Autodesk Inventor part; units mm, degrees
ref_plane "YZ Plane" through (0, 0, 0) normal (1, 0, 0) x (0, 1, 0)
ref_plane "XZ Plane" through (0, 0, 0) normal (0, 1, 0) x (-1, 0, 0)
ref_plane "XY Plane" through (0, 0, 0) normal (0, 0, 1) x (1, 0, 0)
sketch "スケッチ1" plane through (0, 0, 0) normal (0, 0, 1) x (1, 0, 0)
  circle A0 centre (0, 0) radius 25
  dimension "d0" = 50
extrude "押し出し1" add sketch "スケッチ1" along normal blind 15
sketch "スケッチ2" plane through (0, 0, 0) normal (0, 0, -1) x (-1, 0, 0)
  circle A0 centre (0, 0) radius 10
  circle A1 centre (0, 0) radius 21
  dimension "d3" = 20
  dimension "d6" = 42
extrude "押し出し2" cut sketch "スケッチ2" against normal blind 13 contours A0
extrude "押し出し3" cut sketch "スケッチ2" against normal blind 3
chamfer "面取り1" distance 2 angle 45 1 edges at (21, 0, 0)
chamfer "面取り2" distance 2 angle 45 1 edges at (10, 0, 3)
properties part number "storage"
Model file for the job. Use its own axes, mm. A direction names the side the tool comes from. Round coordinates to 2 decimals unless told otherwise and drop trailing zeros. Write each loop counter-clockwise with the first axis right and the second up, starting at its lowest first coordinate (ties: lowest second). Pieces come first, ordered by that corner, then holes. Notation, with made-up numbers: (17, 18.25) -> (29, 18.25) arc R22 ccw to (29, 44.25) -> close; hole circle Ø8 at (19, 74.25). An arc over 180 degrees is marked (long way). Answer as CSV lines item,"result".
1. Pin check, flat tips, straight feed: pin 1 Ø1 at (x, y) = (12, -14) entering from -Z; pin 2 Ø6 at (y, z) = (-10.5, 10.5) entering from +X; pin 3 Ø8 at (y, z) = (19.5, 10) entering from -X. Stop position of each tip, or through.
Resolved:
pin 1,"z = 3"
pin 2,"x = 23.85"
pin 3,"x = -19.62"
2. Slice it at A-A, the plane y = 0. List the corners of the cut face in (x, z).
Resolved:
outline,"(-25, 0) -> (-23, 0) -> (-21, 2) -> (-21, 3) -> (-12, 3) -> (-10, 5) -> (-10, 13) -> (10, 13) -> (10, 5) -> (12, 3) -> (21, 3) -> (21, 2) -> (23, 0) -> (25, 0) -> (25, 15) -> (-25, 15) -> close"
3. Tool access for faces 4 (the face through (0, 0, 15)), 5 (the face through (2.17, -9.76, 8.94)): list every direction of +Z, -Z, +X, -X, +Y, -Y with a clear straight run to the whole face (end or side of a thin tool).
Resolved:
face 4,"+Z, +X, -X, +Y, -Y"
face 5,"-Z"
4. Slice it at C-C, the plane z = 4.25. List the corners of the cut face in (x, y).
Resolved:
outline,"circle Ø50 at (0, 0); hole circle Ø21.5 at (0, 0)"
5. Mould opens along Y. For faces 1 (the face through (-9, -9, 3)), 2 (the face through (22.1, -7.3, 0)), 3 (the face through (23.846, -7.509, 7.395)) say: +Y half, -Y half, draft (parallel to the pull), parting line (faces both ways), or undercut.
Resolved:
face 1,"undercut"
face 2,"draft"
face 3,"parting line"
6. Drill centre lines: line 1 (Y direction, x = 0, z = 10.25); line 2 (Y direction, x = 0, z = 2.3); line 3 (X direction, y = -2, z = 9.5). Where is each one in solid material? Low to high.
Resolved:
line 1,"-25 to -10, 10 to 25"
line 2,"-25 to -21, 21 to 25"
line 3,"-24.92 to -9.8, 9.8 to 24.92"
